```python
from build123d import *

# Parameters (mm, degrees)
ESQUISSE1_R             = 2.9
BOSS_EXTRU_3_DEPTH      = 2
ESQUISSE4_R             = 2.5
BOSS_EXTRU_4_DEPTH      = 1.4
BOSS_EXTRU_5_START      = -13.3
BOSS_EXTRU_5_DEPTH      = 13.3
ESQUISSE6_R             = 3.75
ENL_V_MAT_EXTRU_2_DEPTH = 1
ESQUISSE7_R             = 3.75
ENL_V_MAT_EXTRU_3_DEPTH = 25.863477231
ESQUISSE9_R             = 2.5
ESQUISSE8_R             = 3.65


with BuildPart() as part:
    # Esquisse1 → Boss.-Extru.3 (new body)
    with BuildSketch(Plane.XY):
        with BuildLine():
            Line((-6.65, 8.45), (-6.65, 0))
            Line((-6.65, 0), (6.65, 0))
            Line((6.65, 0), (6.65, 8.45))
            ThreePointArc((6.65, 8.45), (0, 15.1), (-6.65, 8.45))
        make_face()
        with Locations((0, 8.45)):
            Circle(ESQUISSE1_R, mode=Mode.SUBTRACT)
    extrude(amount=-BOSS_EXTRU_3_DEPTH)

    # Esquisse4 → Boss.-Extru.4 (add)
    with BuildSketch(Plane(origin=(0, 0, 0), x_dir=(1, 0, 0), z_dir=(0, 1, 0))):
        with BuildLine():
            Line((6.65, 0), (-6.65, 0))
            Line((-6.65, 0), (-6.65, 12.95))
            ThreePointArc((-6.65, 12.95), (0, 19.6), (6.65, 12.95))
            Line((6.65, 12.95), (6.65, 0))
        make_face()
        with Locations(Location((0, 12.95, 0), (0, 0, 270))):
            Circle(ESQUISSE4_R, mode=Mode.SUBTRACT)
    extrude(amount=BOSS_EXTRU_4_DEPTH)

    # Esquisse5 → Boss.-Extru.5 (add)
    with BuildSketch(Plane.ZY.offset(6.65).offset(BOSS_EXTRU_5_START)):
        with BuildLine():
            Line((-2, 1.4), (-2, 8.3))
            ThreePointArc((-2, 8.3), (-3.599475922, 4.095981854), (-7.2, 1.4))
            Line((-7.2, 1.4), (-2, 1.4))
        make_face()
    extrude(amount=BOSS_EXTRU_5_DEPTH)

    # Esquisse6 → Enlèv. mat.-Extru.2 (cut)
    with BuildSketch(Plane(origin=(0, 0, -2), x_dir=(-1, 0, 0), z_dir=(0, 0, -1))):
        with Locations((0, 8.45)):
            Circle(ESQUISSE6_R)
    extrude(amount=-ENL_V_MAT_EXTRU_2_DEPTH, mode=Mode.SUBTRACT)

    # Esquisse7 → Enlèv. mat.-Extru.3 (cut, through all)
    with BuildSketch(Plane(origin=(0, 0, -1), x_dir=(-1, 0, 0), z_dir=(0, 0, -1))):
        with Locations((0, 8.45)):
            Circle(ESQUISSE7_R)
    extrude(amount=ENL_V_MAT_EXTRU_3_DEPTH, mode=Mode.SUBTRACT)

    # Esquisse9 → Enlèvement de matière-Lissage1 section 0
    with BuildSketch(Plane(origin=(0, 0.4, 0), x_dir=(1, 0, 0), z_dir=(0, 1, 0))):
        with Locations((0, 12.95)):
            Circle(ESQUISSE9_R)
    # Esquisse8 → Enlèvement de matière-Lissage1 section 1
    with BuildSketch(Plane(origin=(0, 1.4, 0), x_dir=(1, 0, 0), z_dir=(0, 1, 0))):
        with Locations((0, 12.95)):
            Circle(ESQUISSE8_R)
    loft(mode=Mode.SUBTRACT)


solid = part.part
```
Can you work these out from the model? Positions are in its coordinate system, mm. A direction names the side the tool comes from. Coordinates: 2 decimals unless noted, no trailing zeros. Loops run counter-clockwise (first coordinate to the right, second up) from the corner with the lowest first, then second, coordinate; pieces in that order, holes last.
1) I need wall thicknesses on probe 1 along X at (y, z) = (0.1, -12.95); probe 2 along X at (y, z) = (8.45, -1.8); probe 3 along Y at (x, z) = (0, -1.7). Which ranges of each line are inside material? Lowest first, please.
2) Thinking about a two-plate mould opening in X: for faces 1 (the flat face through (0, 0, -10)), 2 (the flat face through (-2, 6, -1)), 3 (the cylindrical face through (-0.1, 0.7, -19.6)), 4 (the cylindrical face through (-0.63, 5.62, -0.49)), which applies, pulls with the +X half, pulls with the -X half, needs draft (parallel to the pull), parting line crosses it, or undercut?
3) Imagine slicing it at D-D on y = 9. List the corners of the cut face in (x, z) for me.
4) Imagine slicing it at C-C on x = -5.5. List the corners of the cut face in (y, z) for me.
5) Imagine slicing it at A-A on x = 0. List the corners of the cut face in (y, z) for me, plus the area to 3 significant figures.
6) Imagine slicing it at B-B on y = 7.25. List the corners of the cut face in (x, z) for me, plus the area to 3 significant figures.
7) Which directions (+Z, -Z, +X, -X, +Y, -Y) give clear straight access to the entire face, cutting with the end or side of a thin tool? Please do faces 5 (the flat face through (6.65, 3, -4)), 6 (the cylindrical face through (0.81, 4.79, -1.62)), 7 (the flat face through (2, 1.4, -9)).
8) For pin 1 (5 mm diameter, centred on x = -3.5, z = -2.5, fed in from -Y); pin 2 (5 mm diameter, centred on x = 0, y = 8.45, fed in from -Z); pin 3 (2 mm diameter, centred on x = -1.5, y = 10.5, fed in from -Z); pin 4 (4 mm diameter, centred on x = 5.5, y = 8, fed in from -Z), each with a flat end and sliding along its axis, tell me the tip position at first contact or that it passes through.
Completed:
1. probe 1: x = -6.65 to -2.5, 2.5 to 6.65
1. probe 2: x = -6.65 to -3.75, 3.75 to 6.65
1. probe 3: y = 0 to 4.7, 12.2 to 15.1
2. face 1: needs draft
2. face 2: undercut
2. face 3: parting line crosses it
2. face 4: undercut
3. outline: (-6.63, -2) - (-3.71, -2) - (-3.71, -1) - (-2.85, -1) - (-2.85, 0) - (-6.63, 0) - close; (2.85, -1) - (3.71, -1) - (3.71, -2) - (6.63, -2) - (6.63, 0) - (2.85, 0) - close
4. outline: (0, -16.69) - (1.4, -16.69) - (1.4, -7.2) arc R8.07 cw to (8.3, -2) - (12.19, -2) - (12.19, 0) - (0, 0) - close
5. outline: (0, -19.6) - (1.4, -19.6) - (1.4, -16.6) - (0.4, -15.45) - (0, -15.45) - close; (0, -10.45) - (0.4, -10.45) - (1.4, -9.3) - (1.4, -7.2) arc R8.07 cw to (4.7, -3.19) - (4.7, -1) - (5.55, -1) - (5.55, 0) - (0, 0) - close; (11.35, -1) - (12.2, -1) - (12.2, -2) - (15.1, -2) - (15.1, 0) - (11.35, 0) - close
5. area: 42.4 mm2
6. outline: (-6.65, -2.16) - (-3.55, -2.16) - (-3.55, -1) - (-2.64, -1) - (-2.64, 0) - (-6.65, 0) - close; (2.64, -1) - (3.55, -1) - (3.55, -2.16) - (6.65, -2.16) - (6.65, 0) - (2.64, 0) - close
6. area: 15.2 mm2
7. face 5: +Z, -Z, +X, +Y, -Y
7. face 6: -Z
7. face 7: -Z, +X, -X, +Y
8. pin 1: stops at y = 0
8. pin 2: passes through
8. pin 3: stops at z = -1
8. pin 4: stops at z = -2.53
